Read the model definition and answer for the solid it produces. Units are mm, in the model's axes. Coordinates: 2 decimals unless noted, no trailing zeros. Write each loop counter-clockwise with the first axis right and the second up, starting at its lowest first coordinate (ties: lowest second). Pieces come first, ordered by that corner, then holes. Notation, with made-up numbers: (56.5, 12) -> (114.5, 12) arc R25 cw to (114.5, 28) -> close; hole circle Ø11 at (66.5, 11). An arc over 180 degrees is marked (long way). Use CSV: the item, a comma, the result in double quotes.
from build123d import *

# Parameters (mm, degrees)
SKETCH1_W           = 22.5
SKETCH1_H           = 15
BOSS_EXTRUDE1_DEPTH = 0.5
WRAP1_OUTLINE_W     = 0.826388889
WRAP1_OUTLINE_H     = 3.5
WRAP1_DEPTH         = 0.5


# Read off the part's stored shape, not the designer's step: Wrap1
with BuildPart() as part:
    # Sketch1 → Boss-Extrude1 (new body)
    with BuildSketch(Plane.XY):
        Rectangle(SKETCH1_W, SKETCH1_H)
    extrude(amount=BOSS_EXTRUDE1_DEPTH)

    # Wrap1 outline → Wrap1 (add)
    # profile 1 of 4: a face of its own
    with BuildSketch(Plane.XY.offset(0.5)):
        with BuildLine():
            add(Edge.make_bspline(
                [(2.118055556, -1.8), (2.102101425, -1.731019264), (2.069534878, -1.59021157), (2.021189223, -1.454006194), (1.996527778, -1.38452691)],
                knots=[0, 0, 0, 0, 0.489893232, 1, 1, 1, 1], degree=3))
            Line((2.118055556, -1.8), (2.506944444, -1.8))
            Line((2.506944444, -1.8), (2.506944444, 0.047222222))
            Line((2.506944444, 0.047222222), (1.097222222, 0.047222222))
            Line((1.097222222, 0.047222222), (1.097222222, -0.584722222))
            Line((1.097222222, -0.584722222), (1.729166667, -0.584722222))
            add(Edge.make_bspline(
                [(1.189887153, -1.168055556), (1.224007135, -1.166641415), (1.291557812, -1.163841703), (1.389411618, -1.135479706), (1.48186011, -1.091912059), (1.552522736, -1.041311507), (1.604163451, -0.992684417), (1.637831654, -0.949615289), (1.665872255, -0.901112075), (1.689666798, -0.848077449), (1.70692943, -0.789214567), (1.719447815, -0.72564884), (1.728419327, -0.65687553), (1.728911975, -0.609311898), (1.729166667, -0.584722222)],
                knots=[0, 0, 0, 0, 0.113839351, 0.225378937, 0.337862557, 0.454399889, 0.514282548, 0.574582762, 0.636443988, 0.701264893, 0.768496234, 0.841060889, 0.917830892, 1, 1, 1, 1], degree=3))
            add(Edge.make_bspline(
                [(0.513888889, -0.076584201), (0.514572313, -0.119635576), (0.515896024, -0.203021042), (0.523217979, -0.32423507), (0.536468218, -0.437450039), (0.556814389, -0.542753882), (0.58016669, -0.640850258), (0.610908424, -0.730891969), (0.646278395, -0.813189447), (0.687302005, -0.887392166), (0.733771509, -0.953045942), (0.784892562, -1.010472833), (0.840544687, -1.059907744), (0.901681039, -1.099399842), (0.967335449, -1.130329733), (1.037327541, -1.152255059), (1.112172234, -1.165456245), (1.163501396, -1.167173038), (1.189887153, -1.168055556)],
                knots=[0, 0, 0, 0, 0.089605155, 0.173554681, 0.252640076, 0.326637626, 0.396673525, 0.462328207, 0.524393538, 0.582893738, 0.638453156, 0.691446992, 0.742603933, 0.792882167, 0.842383995, 0.893214225, 0.945106771, 1, 1, 1, 1], degree=3))
            add(Edge.make_bspline(
                [(1.155707465, 1.068055556), (1.130075838, 1.067210899), (1.079949494, 1.065559051), (1.00696703, 1.051696413), (0.938909467, 1.028085171), (0.875814409, 0.994871993), (0.817591808, 0.952846932), (0.76484425, 0.901059239), (0.716596885, 0.840386196), (0.673656251, 0.770352319), (0.635825562, 0.691866233), (0.603288773, 0.605321415), (0.575274497, 0.511186428), (0.552534046, 0.408895639), (0.535554331, 0.298727159), (0.522524141, 0.180656658), (0.514960566, 0.054664626), (0.514252816, -0.03201382), (0.513888889, -0.076584201)],
                knots=[0, 0, 0, 0, 0.052392573, 0.102461232, 0.15126336, 0.199209074, 0.247788165, 0.29759102, 0.349914456, 0.405956949, 0.465245134, 0.527852777, 0.594860669, 0.665966982, 0.741990387, 0.822734633, 0.908849485, 1, 1, 1, 1], degree=3))
            add(Edge.make_bspline(
                [(1.729166667, 0.436111111), (1.725153755, 0.461736316), (1.717367072, 0.511459652), (1.701192738, 0.583185082), (1.6824977, 0.649991098), (1.660322693, 0.711876638), (1.635538667, 0.768921126), (1.607174662, 0.820915366), (1.576291477, 0.868236988), (1.541672833, 0.910237935), (1.50458923, 0.948097333), (1.463146746, 0.97958563), (1.419810775, 1.00755935), (1.372711281, 1.02959383), (1.322861274, 1.047089034), (1.269581929, 1.059092439), (1.213672152, 1.066996713), (1.175230511, 1.067698927), (1.155707465, 1.068055556)],
                knots=[0, 0, 0, 0, 0.082191489, 0.159484973, 0.232898467, 0.301940512, 0.367695662, 0.429819924, 0.48946921, 0.54649677, 0.602106423, 0.65700512, 0.711106214, 0.765308393, 0.821396578, 0.878237506, 0.938161464, 1, 1, 1, 1], degree=3))
            Line((1.729166667, 0.436111111), (2.506944444, 0.537890625))
            add(Edge.make_bspline(
                [(1.13671875, 1.748611111), (1.183852349, 1.747570689), (1.276092384, 1.745534592), (1.411034443, 1.730174961), (1.539027431, 1.704764538), (1.659857093, 1.667729236), (1.774225525, 1.621890079), (1.880970414, 1.564492815), (1.980736808, 1.497041103), (2.072943296, 1.419502923), (2.158223008, 1.333869175), (2.234134407, 1.240180481), (2.301231448, 1.13974161), (2.361087022, 1.033221224), (2.410889646, 0.919073074), (2.452005017, 0.798088035), (2.484825247, 0.670596043), (2.499495457, 0.582581264), (2.506944444, 0.537890625)],
                knots=[0, 0, 0, 0, 0.070069074, 0.137124556, 0.201650146, 0.263813257, 0.324771258, 0.384560312, 0.443656803, 0.503520473, 0.563413726, 0.623088901, 0.682497508, 0.742828077, 0.80451978, 0.867376611, 0.932658764, 1, 1, 1, 1], degree=3))
            add(Edge.make_bspline(
                [(-0.361111111, -0.097092014), (-0.360056629, -0.029193424), (-0.357998366, 0.103338977), (-0.338716764, 0.296809121), (-0.30692414, 0.479850097), (-0.262920099, 0.652858131), (-0.207057789, 0.816068001), (-0.137589586, 0.968937488), (-0.055342885, 1.111319656), (0.038529131, 1.243069192), (0.144049567, 1.361084804), (0.258050156, 1.46596394), (0.383121972, 1.552519732), (0.516042062, 1.624841653), (0.658464001, 1.680557916), (0.809966935, 1.71955882), (0.970283346, 1.744948697), (1.080412506, 1.747372091), (1.13671875, 1.748611111)],
                knots=[0, 0, 0, 0, 0.076094269, 0.148529686, 0.217678594, 0.284172559, 0.348435986, 0.410796815, 0.472084106, 0.532492434, 0.591791888, 0.649255708, 0.705707708, 0.761835604, 0.81854385, 0.876643326, 0.936930864, 1, 1, 1, 1], degree=3))
            add(Edge.make_bspline(
                [(1.059244792, -1.848611111), (1.004723071, -1.847238309), (0.89821979, -1.844556663), (0.743173288, -1.821117291), (0.597057137, -1.783836147), (0.461013751, -1.729005295), (0.333422729, -1.660627785), (0.216232156, -1.575256979), (0.107153099, -1.476073515), (0.009896653, -1.360905337), (-0.076894112, -1.234286084), (-0.153291075, -1.098351542), (-0.218137905, -0.953529332), (-0.27026294, -0.799278052), (-0.311528227, -0.636281671), (-0.339716794, -0.464234977), (-0.35768967, -0.28356275), (-0.359953571, -0.160178706), (-0.361111111, -0.097092014)],
                knots=[0, 0, 0, 0, 0.064345405, 0.125692964, 0.184718006, 0.242009577, 0.298461161, 0.355213548, 0.412768934, 0.472141974, 0.532760404, 0.593797592, 0.656024627, 0.719840029, 0.785822383, 0.854335256, 0.925521109, 1, 1, 1, 1], degree=3))
            add(Edge.make_bspline(
                [(1.996527778, -1.38452691), (1.965683846, -1.421481302), (1.905191378, -1.493957872), (1.802494662, -1.587913316), (1.69486425, -1.668972518), (1.580037705, -1.734766305), (1.458573377, -1.785831157), (1.330913621, -1.822576666), (1.196939841, -1.844019509), (1.105653567, -1.847063556), (1.059244792, -1.848611111)],
                knots=[0, 0, 0, 0, 0.133004575, 0.260854394, 0.383963685, 0.505044677, 0.625870246, 0.747551188, 0.871658247, 1, 1, 1, 1], degree=3))
        make_face()
    # profile 2 of 4: a face of its own
    with BuildSketch(Plane.XY.offset(0.5)):
        Polygon((-2.111111111, -1.8), (-2.111111111, -1.119444444), (-3.520833333, -1.119444444), (-3.520833333, 1.7), (-4.347222222, 1.7), (-4.347222222, -1.8), align=None)
    # profile 3 of 4: a face of its own
    with BuildSketch(Plane.XY.offset(0.5)):
        with Locations((-1.309027778, -0.05)):
            Rectangle(WRAP1_OUTLINE_W, WRAP1_OUTLINE_H)
    # profile 4 of 4: a face of its own
    with BuildSketch(Plane.XY.offset(0.5)):
        Polygon((5.076497396, -1.8), (5.958333333, -1.8), (4.885850694, 1.7), (3.880208333, 1.7), (2.798611111, -1.8), (3.516384549, -1.8), (3.731336806, -1.070833333), (4.853190104, -1.070833333), align=None)
        Polygon((4.28125, 0.795377604), (4.659505208, -0.438888889), (3.917426215, -0.438888889), align=None, mode=Mode.SUBTRACT)
    extrude(amount=WRAP1_DEPTH)


solid = part.part
1. Find the intervals of material crossed by line 1 along Y through (x, z) = (0.75, 0.55); line 2 along Z through (x, y) = (-10, 6.25); line 3 along Y through (x, z) = (0, 0.75), in increasing order.
Solutions:
line 1,"y = -1.82 to -0.97, 0.88 to 1.7"
line 2,"z = 0 to 0.5"
line 3,"y = -1.34 to 1.19"
2. A cutting plane is placed at B-B (x = -3.25). Give the vertices of the cut face in (y, z), and give its area (3 significant figures).
Solutions:
outline,"(-7.5, 0) -> (7.5, 0) -> (7.5, 0.5) -> (-1.12, 0.5) -> (-1.12, 1) -> (-1.8, 1) -> (-1.8, 0.5) -> (-7.5, 0.5) -> close"
area,"7.84 mm^2"
3. For a pull along X with two mould halves and no side action, classify faces 1 (the flat face through (5.43, -0.07, 0.75)), 2 (the flat face through (5, 0, 1)), 3 (the flat face through (3.347, -0.026, 0.746)) as pulls with the +X half, pulls with the -X half, needs draft (parallel to the pull), parting line crosses it, or undercut.
Solutions:
face 1,"pulls with the +X half"
face 2,"needs draft"
face 3,"undercut"
4. Each of these flat-tipped pins is pushed along its axis until it touches: pin 1 Ø0.6 at (x, z) = (-1.5, 1) entering from +Y; pin 2 Ø0.6 at (x, z) = (5.5, 1) entering from -Y. Where does it stop, or does it pass through?
Solutions:
pin 1,"stops at y = 1.7"
pin 2,"stops at y = -1.8"
5. A cutting plane is placed at D-D (x = 9.75). Give the vertices of the cut face in (y, z), and give its area (3 significant figures).
Solutions:
outline,"(-7.5, 0) -> (7.5, 0) -> (7.5, 0.5) -> (-7.5, 0.5) -> close"
area,"7.50 mm^2"
6. A cutting plane is placed at A-A (z = 0.7). Give the number of separate pieces and of enclosed holes in the cut face, and give its area (3 significant figures).
Solutions:
separate pieces,"4"
enclosed holes,"1"
area,"19.1 mm^2"
7. A cutting plane is placed at C-C (y = 4.75). Give the vertices of the cut face in (x, z), and give its area (4 significant figures).
Solutions:
outline,"(-11.25, 0) -> (11.25, 0) -> (11.25, 0.5) -> (-11.25, 0.5) -> close"
area,"11.25 mm^2"
